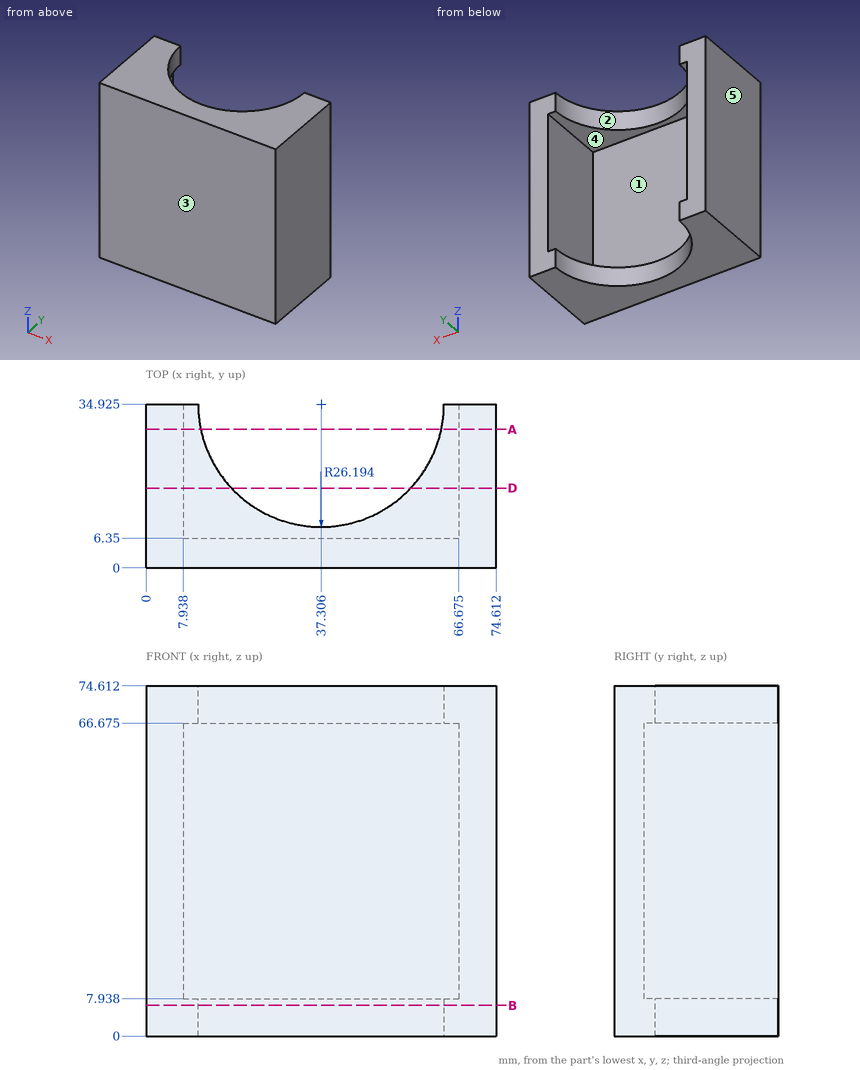
Drawing for the job (mm, zero at the part's lowest x, y, z). A direction names the side the tool comes from. Coordinates: 2 decimals unless noted, no trailing zeros. Order: outer loops, then holes, each group sorted by start corner. A loop starts at its lowest first (then second) coordinate and runs counter-clockwise, first axis right, second up. Notation, with made-up numbers: (17.25, 23.5) - (46.25, 23.5) arc R25 ccw to (46.25, 47.5) - close; hole circle Ø10 at (-27, -15.5). An arc over 180 degrees is marked (long way). Use a Markdown table: item, result. Add a question column.
(1) Saw through at B-B (z = 6.5). Give the cut face in (x, y) (1 decimal).
(2) Which spindle directions (+Z, -Z, +X, -X, +Y, -Y) get a long thin tool onto all of the face, cutting with end or side? Do the marked faces 1 and 2. Say none if no direction does.
(3) Saw through at A-A (y = 29.5). Give the cut face in (x, z) (1 decimal), then the cut area to 3 significant figures.
(4) Pull direction X, two halves, no side cores. Call the marked faces 3, 4 and 5: +X half, -X half, draft (parallel to the pull), parting line (faces both ways), or undercut.
(5) Saw through at D-D (y = 17). Give the cut face in (x, z) (1 decimal).
(6) Flat gauge pins, fed straight in: pin 1 (8.5 mm diameter, centred on x = 31.5, y = 14.5, fed in from -Z); pin 2 (12 mm diameter, centred on x = 22.5, z = 45, fed in from +Y). Where does each tip first touch, or does it go through?
(7) Drill centre lines: line 1 along X through (y, z) = (30, 42) (1 decimal); line 2 along Y through (x, z) = (17, 28). Where is each one in solid material? Low to high. Write a range as [from, to].
Solved:
| question | item | result |
|---|---|---|
| 1 | outline | (0, 0) - (74.6, 0) - (74.6, 34.9) - (63.5, 34.9) arc R26.2 cw to (11.1, 34.9) - (0, 34.9) - close |
| 2 | face 1 | +Y |
| 2 | face 2 | +Z, -Z, +Y |
| 3 | outline | (0, 0) - (11.7, 0) - (11.7, 7.9) - (7.9, 7.9) - (7.9, 66.7) - (11.7, 66.7) - (11.7, 74.6) - (0, 74.6) - close; (62.9, 0) - (74.6, 0) - (74.6, 74.6) - (62.9, 74.6) - (62.9, 66.7) - (66.7, 66.7) - (66.7, 7.9) - (62.9, 7.9) - close |
| 3 | area | 1,300 mm² |
| 4 | face 3 | draft |
| 4 | face 4 | undercut |
| 4 | face 5 | -X half |
| 5 | outline | (0, 0) - (18.2, 0) - (18.2, 7.9) - (7.9, 7.9) - (7.9, 66.7) - (18.2, 66.7) - (18.2, 74.6) - (0, 74.6) - close; (56.4, 0) - (74.6, 0) - (74.6, 74.6) - (56.4, 74.6) - (56.4, 66.7) - (66.7, 66.7) - (66.7, 7.9) - (56.4, 7.9) - close |
| 6 | pin 1 | passes through |
| 6 | pin 2 | stops at y = 6.35 |
| 7 | line 1 | x = [0, 7.9], [66.7, 74.6] |
| 7 | line 2 | y = [0, 6.35] |
